from build123d import *

# Parameters (mm, degrees)
SKETCH1_W           = 82.7
SKETCH1_H           = 71
BOSS_EXTRUDE1_DEPTH = 5
SKETCH3_W           = 25
SKETCH3_H           = 5
SKETCH3_W_2         = 5
SKETCH3_H_2         = 25
BOSS_EXTRUDE2_DEPTH = 5
SKETCH4_R           = 2
CUT_EXTRUDE1_DEPTH  = 5
SKETCH5_R           = 4
SKETCH5_R_2         = 2
BOSS_EXTRUDE3_DEPTH = 5


with BuildPart() as part:
    # Sketch1 → Boss-Extrude1 (new body)
    with BuildSketch(Plane.XY):
        Rectangle(SKETCH1_W, SKETCH1_H)
    extrude(amount=BOSS_EXTRUDE1_DEPTH)

    # Sketch3 → Boss-Extrude2 (add)
    with BuildSketch(Plane.XY.offset(5)):
        with Locations((0, 38)):
            Rectangle(SKETCH3_W, SKETCH3_H)
        with Locations((43.85, 0)):
            Rectangle(SKETCH3_W_2, SKETCH3_H_2)
        with Locations((0, -38)):
            Rectangle(SKETCH3_W, SKETCH3_H)
    extrude(amount=-BOSS_EXTRUDE2_DEPTH)

    # Sketch4 → Cut-Extrude1 (cut)
    with BuildSketch(Plane.XY.offset(5)):
        with Locations((0, 38)):
            Circle(SKETCH4_R)
        with Locations((0, -38)):
            Circle(SKETCH4_R)
    extrude(amount=-CUT_EXTRUDE1_DEPTH, mode=Mode.SUBTRACT)

    # Sketch5 → Boss-Extrude3 (add)
    # profile 1 of 2: a face of its own
    with BuildSketch(Plane.XY.offset(5)):
        with Locations((0, 38)):
            Circle(SKETCH5_R)
        with Locations((0, 38)):
            Circle(SKETCH5_R_2, mode=Mode.SUBTRACT)
    # profile 2 of 2: a face of its own
    with BuildSketch(Plane.XY.offset(5)):
        with Locations((0, -38)):
            Circle(SKETCH5_R)
        with Locations((0, -38)):
            Circle(SKETCH5_R_2, mode=Mode.SUBTRACT)
    extrude(amount=-BOSS_EXTRUDE3_DEPTH)


solid = part.part
Model file for the job. Use its own axes, mm. A direction names the side the tool comes from. Coordinates: 2 decimals unless noted, no trailing zeros. Write each loop counter-clockwise with the first axis right and the second up, starting at its lowest first coordinate (ties: lowest second). Pieces come first, ordered by that corner, then holes. Notation, with made-up numbers: (83.25, 37) -> (89.25, 37) arc R17 ccw to (89.25, 45) -> close; hole circle Ø10 at (25, 33). An arc over 180 degrees is marked (long way). One line per item, written item: value. Start each with the question number.
1) Pull direction X, two halves, no side cores. Call faces 4 (the face through (2, 1, 0)), 5 (the face through (0, 36, 3)), 6 (the face through (0, -40, 3)), 7 (the face through (12.5, -38, 3)): +X half, -X half, draft (parallel to the pull), parting line (faces both ways), or undercut.
2) Probe probe 1 along Y at (x, z) = (0, 1.6); probe 2 along Y at (x, z) = (28, 4.7); probe 3 along X at (y, z) = (21.5, 4.55). List the from-to ranges inside material, lowest first.
3) Slice it at D-D on x = -26.5. Write the cut outline in (y, z).
4) Flat gauge pins, fed straight in: pin 1 Ø2 at (x, z) = (28, 4) entering from -Y; pin 2 Ø2 at (y, z) = (30.5, 2.5) entering from +X; pin 3 Ø1 at (x, z) = (9, 2) entering from -Y. Where does each tip first touch, or does it go through?
5) Slice it at B-B on z = 1.2. Write the cut outline in (x, y), then the cut area to 3 significant figures.
6) Slice it at A-A on y = -38. Write the cut outline in (x, z), then the cut area to 3 significant figures.
7) Which spindle directions (+Z, -Z, +X, -X, +Y, -Y) get a long thin tool onto all of the face, cutting with end or side? Do faces 1 (the face through (27, -35.5, 2)), 2 (the face through (-8, 40.5, 3)), 3 (the face through (8, 40.5, 3)). Say none if no direction does.
8) Slice it at C-C on x = 0. Write the cut outline in (y, z), then the cut area to 3 significant figures.
Answers follow:
1. face 4: draft
1. face 5: undercut
1. face 6: undercut
1. face 7: +X half
2. probe 1: -42 to -40, -36 to 36, 40 to 42
2. probe 2: -35.5 to 35.5
2. probe 3: -41.35 to 41.35
3. outline: (-35.5, 0) -> (35.5, 0) -> (35.5, 5) -> (-35.5, 5) -> close
4. pin 1: y = -35.5
4. pin 2: x = 41.35
4. pin 3: y = -40.5
5. outline: (-41.35, -35.5) -> (-12.5, -35.5) -> (-12.5, -40.5) -> (-3.12, -40.5) arc R4 ccw to (3.12, -40.5) -> (12.5, -40.5) -> (12.5, -35.5) -> (41.35, -35.5) -> (41.35, -12.5) -> (46.35, -12.5) -> (46.35, 12.5) -> (41.35, 12.5) -> (41.35, 35.5) -> (12.5, 35.5) -> (12.5, 40.5) -> (3.12, 40.5) arc R4 ccw to (-3.12, 40.5) -> (-12.5, 40.5) -> (-12.5, 35.5) -> (-41.35, 35.5) -> close; hole circle Ø4 at (0, -38); hole circle Ø4 at (0, 38)
5. area: 6,230 mm2
6. outline: (-12.5, 0) -> (-2, 0) -> (-2, 5) -> (-12.5, 5) -> close; (2, 0) -> (12.5, 0) -> (12.5, 5) -> (2, 5) -> close
6. area: 105 mm2
7. face 1: +Z, -Z, +X, -Y
7. face 2: +Z, -Z, -X, +Y
7. face 3: +Z, -Z, +X, +Y
8. outline: (-42, 0) -> (-40, 0) -> (-40, 5) -> (-42, 5) -> close; (-36, 0) -> (36, 0) -> (36, 5) -> (-36, 5) -> close; (40, 0) -> (42, 0) -> (42, 5) -> (40, 5) -> close
8. area: 380 mm2
